For this review, use the dimensioned drawing (mm, ordinates from the lowest corner) and the shaded views. A direction names the side the tool comes from. Round coordinates to 2 decimals unless told otherwise and drop trailing zeros. Loops run counter-clockwise (first coordinate to the right, second up) from the corner with the lowest first, then second, coordinate; pieces in that order, holes last. Notation, with made-up numbers: M 35.25,15.25 L 54.25,15.25 A21 cw 54.25,46.25 Z; hole C 31,-4.5 d8. An arc over 180 degrees is marked long. Use a Markdown table: item, result. Add a question column.
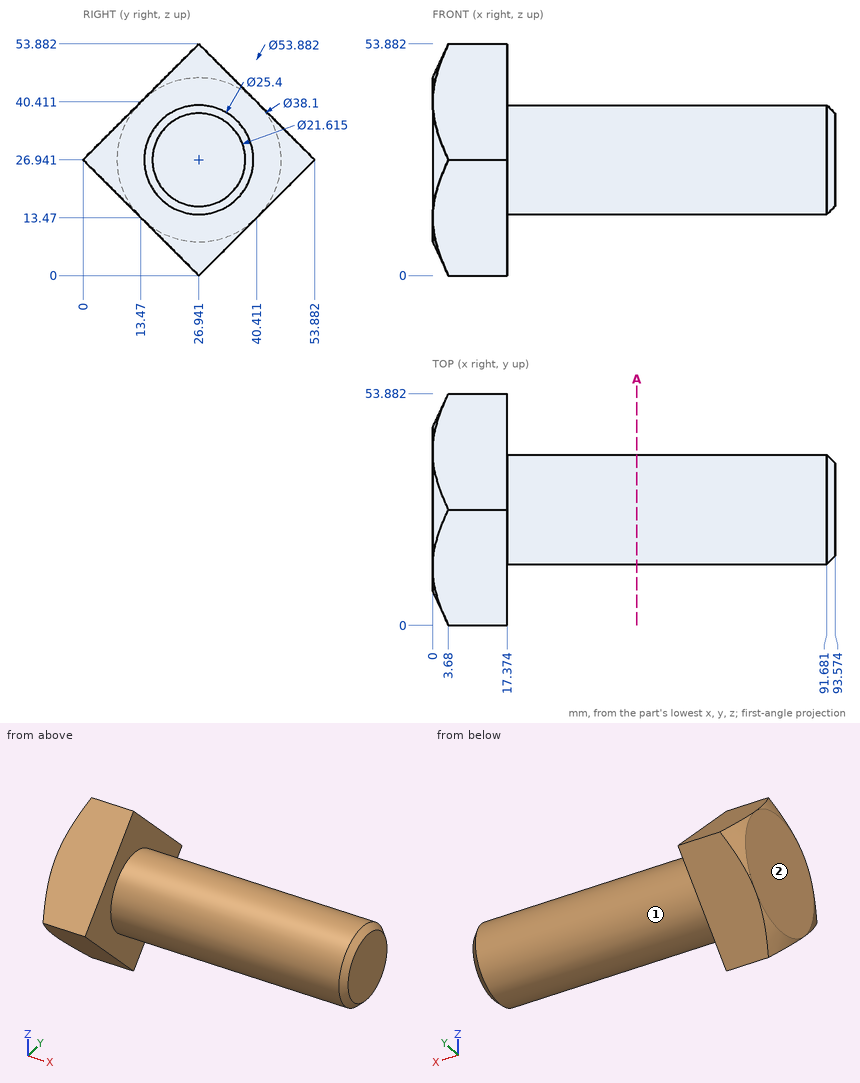
(1) Insertion check: pin 1 Ø3 at (x, y) = (17, 11) entering from +Z; pin 2 Ø2 at (x, y) = (46, 12.5) entering from +Z (3 decimals); pin 3 Ø3 at (x, z) = (29, 14.5) entering from +Y; pin 4 Ø6 at (x, z) = (13.5, 31) entering from -Y. Each pin has a flat end and moves straight along its axis. Give the tip position at first contact, or say it passes through.
(2) For the marked faces 1 and 2, list the 3-axis set-ups (+Z, -Z, +X, -X, +Y, -Y) from which the entire face can be reached by the end or side of a thin tool; tool diameter is ignored.
(3) To check wall thickness, follow probe 1 along X at (y, z) = (18.5, 12); probe 2 along Z at (x, y) = (76.5, 28.5) (1 decimal); probe 3 along Z at (x, y) = (54.5, 26) (1 decimal). State the ranges of each line that lie inside material, in increasing order.
(4) Consider section A-A, the plane x = 47.5. Give the boundary of the cut face in (y, z).
Found:
| question | item | result |
|---|---|---|
| 1 | pin 1 | stops at z = 39.44 |
| 1 | pin 2 | passes through |
| 1 | pin 3 | stops at y = 33.39 |
| 1 | pin 4 | stops at y = 1.06 |
| 2 | face 1 | +X |
| 2 | face 2 | +Z, -Z, -X, +Y, -Y |
| 3 | probe 1 | x = 0 to 17.37 |
| 3 | probe 2 | z = 14.3 to 39.5 |
| 3 | probe 3 | z = 14.3 to 39.6 |
| 4 | outline | C 26.94,26.94 d25.4 |
